Input: dimensioned drawing with shaded views. Units: mm. Origin: part minimum x, y, z. Coordinates: 2 decimals unless noted, no trailing zeros. Order: outer loops, then holes, each group sorted by start corner. A loop starts at its lowest first (then second) coordinate and runs counter-clockwise, first axis right, second up. Notation, with made-up numbers: (62, 55) -> (87, 55) arc R10 cw to (87, 71) -> close; hole circle Ø5 at (-36.5, 0.5). An arc over 180 degrees is marked (long way). Answer as CSV lines item,"result".
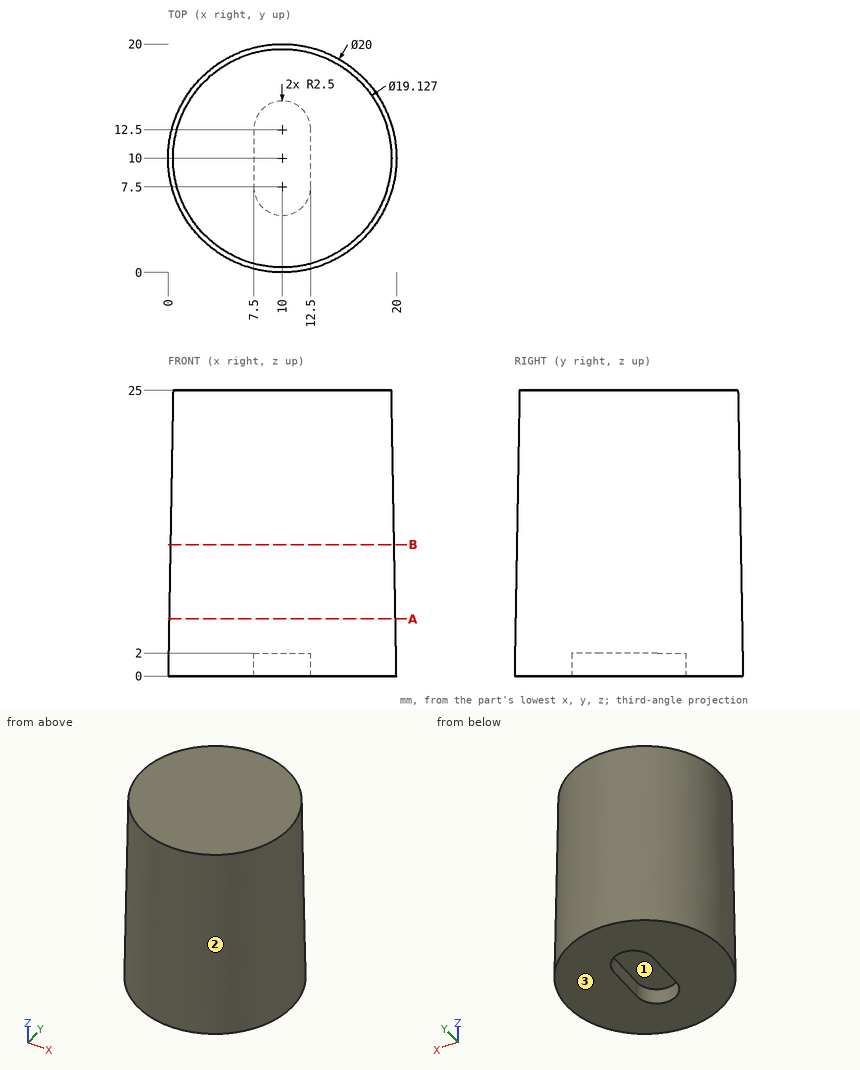
1. Contact query for flat-ended pins moving along their axis: pin 1 (10 mm diameter, centred on y = 6.5, z = 13.5, fed in from -X); pin 2 (2.5 mm diameter, centred on x = 10, y = 9.5, fed in from -Z); pin 3 (2 mm diameter, centred on x = 12.5, z = 3.5, fed in from +Y). Output: stop coordinate, or through.
Findings:
pin 1,"stops at x = 0.17"
pin 2,"stops at z = 2"
pin 3,"stops at y = 19.83"
2. Cut plane B-B (z = 11.5). Return the cut outline in (x, y), plus the area to 3 significant figures.
Findings:
outline,"circle Ø19.6 at (10, 10)"
area,"302 mm2"
3. Cut plane A-A (z = 5). Return the cut outline in (x, y) (1 decimal), plus the area to 3 significant figures.
Findings:
outline,"circle Ø19.8 at (10, 10)"
area,"309 mm2"
4. Mould query, pull axis Y, two halves, no side actions, for the marked faces 1, 2 and 3. Classes: released by +Y, released by -Y, zero draft, split by the parting line, or undercut.
Findings:
face 1,"undercut"
face 2,"split by the parting line"
face 3,"zero draft"
5. Ray query, line 1 along X through (y, z) = (12.5, 1.5) (1 decimal); line 2 along Z through (x, y) = (8.25, 9.25); line 3 along X through (y, z) = (13.75, 19.25). Return the intervals inside material, ascending.
Findings:
line 1,"x = 0.3 to 7.5, 12.5 to 19.7"
line 2,"z = 2 to 25"
line 3,"x = 1.09 to 18.91"
